Read the model definition and answer for the solid it produces. Units are mm, in the model's axes. Face numbers are marked on the shaded views. Round coordinates to 2 decimals unless told otherwise and drop trailing zeros. Write each loop counter-clockwise with the first axis right and the second up, starting at its lowest first coordinate (ties: lowest second). Pieces come first, ordered by that corner, then holes.
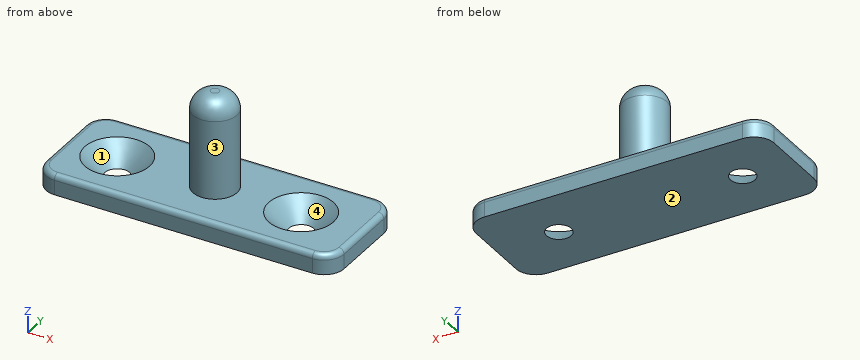
from build123d import *

# Parameters (mm, degrees)
F0_R     = 2.794
F1_DEPTH = 14.732
F0_W     = 37.719
F0_H     = 13.6906
F0_R_2   = 1.5621
F2_DEPTH = 2.54
F3_SIZE  = 2.53999
F4_R     = 2.54
F5_R     = 2.2688779059
F6_R     = 0.6745312693


# Not quite as in the source:
# - a fillet or chamfer is up to 0.001 mm smaller than in the source, because OpenCascade refuses the exact size


with BuildPart() as f1:
    # F0 (on Top) → F1 (new body)
    with BuildSketch(Plane.XY):
        Circle(F0_R)
    extrude(amount=F1_DEPTH)

    # F0 (on Top) → F2 (join)
    with BuildSketch(Plane.XY):
        Rectangle(F0_W, F0_H)
        with Locations((-12.3765456688, 0)):
            Circle(F0_R_2, mode=Mode.SUBTRACT)
        Circle(F0_R, mode=Mode.SUBTRACT)
        with Locations((10.9031473519, 0)):
            Circle(F0_R_2, mode=Mode.SUBTRACT)
    extrude(amount=F2_DEPTH)

    # F3 (size 2.54 in the source; OpenCascade refuses exactly that, so slightly less here)
    f3_edges = [f1.edges().sort_by_distance(p)[0] for p in [
        (-13.938646, 0, 2.54),
        (9.341047, 0, 2.54),
    ]]
    chamfer(f3_edges, length=F3_SIZE)

    # F4
    f4_edges = [f1.edges().sort_by_distance(p)[0] for p in [
        (18.8595, -6.8453, 1.27),
        (18.8595, 6.8453, 1.27),
        (-18.8595, -6.8453, 1.27),
        (-18.8595, 6.8453, 1.27),
    ]]
    fillet(f4_edges, radius=F4_R)

    # F5
    f5_edges = [f1.edges().sort_by_distance(p)[0] for p in [
        (-2.794, 0, 14.732),
    ]]
    fillet(f5_edges, radius=F5_R)

    # F6
    f6_edges = [f1.edges().sort_by_distance(p)[0] for p in [
        (0, -6.8453, 2.54),
        (18.115551, -6.101351, 2.54),
        (18.8595, 0, 2.54),
        (0, 6.8453, 2.54),
        (18.115551, 6.101351, 2.54),
        (-18.115551, 6.101351, 2.54),
        (-18.8595, 0, 2.54),
        (-18.115551, -6.101351, 2.54),
    ]]
    fillet(f6_edges, radius=F6_R)


solid = f1.part
Q1. Section A-A (y = 0) is taken. State how many separate pieces and enclosed holes the cut face has, then the cut area to 3 significant figures.
Verdict:
separate pieces: 3
enclosed holes: 0
area: 133 mm2
Q2. Flat-ended cylindrical pins translate along their axes: pin 1 Ø5 at (x, z) = (3.5, 8.5) entering from -Y; pin 2 Ø5 at (y, z) = (4.5, 12) entering from -X; pin 3 Ø3 at (x, y) = (-12.38, 0) entering from -Z; pin 4 Ø2 at (y, z) = (0, 4) entering from -X. Find the tip coordinate at first contact, or state that the pin passes through.
Verdict:
pin 1: stops at y = -2.61
pin 2: stops at x = -1.95
pin 3: passes through
pin 4: stops at x = -2.79
Q3. Section B-B (z = 3.5) is taken. Determine the outline of the cut face in (x, y).
Verdict:
outline: circle Ø5.59 at (0, 0)
Q4. Straight lines are drawn through the part: probe 1 along X at (y, z) = (0, 0.05); probe 2 along X at (y, z) = (2, 1.5); probe 3 along Z at (x, y) = (-8.5, 5.5). For each, find the intervals that lie inside material, in ascending order.
Verdict:
probe 1: x = -18.86 to -13.99, -10.76 to 9.29, 12.52 to 18.86
probe 2: x = -18.86 to -14.7, -10.06 to 8.58, 13.22 to 18.86
probe 3: z = 0 to 2.54
Q5. Determine the mould class of the marked faces 1, 2, 3 and 4 for opening direction Y: pulls with the +Y half, pulls with the -Y half, needs draft (parallel to the pull), parting line crosses it, or undercut.
Verdict:
face 1: undercut
face 2: needs draft
face 3: parting line crosses it
face 4: undercut
